Design review of the part built by this model. Coordinates are the model's own, in mm. Coordinates: 2 decimals unless noted, no trailing zeros. Loops run counter-clockwise (first coordinate to the right, second up) from the corner with the lowest first, then second, coordinate; pieces in that order, holes last. Notation, with made-up numbers: M 27,3.5 L 70,3.5 A17 cw 70,12.5 Z; hole C -33.5,19 d4. An arc over 180 degrees is marked long. One line per item, written item: value.
```python
from build123d import *

# Parameters (mm, degrees)
BASE_FLANGE1_DEPTH           = 3.175
SKETCH8_W                    = 12.7
SKETCH8_H                    = 3.175
CUT_EXTRUDE2_DEPTH           = 309.926847379
SKETCH11_R                   = 3.175
CUT_EXTRUDE4_DEPTH           = 309.926847379
SKETCH21_R                   = 2.5527
CUT_EXTRUDE5_DEPTH           = 309.926847379
SKETCH23_W                   = 25.4
SKETCH23_H                   = 3.175
TAB1_DEPTH                   = 3.175
CSK_FOR_M3_SFHCS1_AT_2_COUNT = 2
CSK_FOR_M3_SFHCS1_AT_2_PITCH = 16
CSK_FOR_M3_SFHCS1_AT_3_COUNT = 2
CSK_FOR_M3_SFHCS1_AT_3_PITCH = 27.712812921
CSK_FOR_M3_SFHCS1_AT_4_COUNT = 2
CSK_FOR_M3_SFHCS1_AT_4_PITCH = 32
CSK_FOR_M3_SFHCS1_AT_5_COUNT = 2
CSK_FOR_M3_SFHCS1_AT_5_PITCH = 27.712812921
CSK_FOR_M3_SFHCS1_AT_6_COUNT = 2
CSK_FOR_M3_SFHCS1_AT_6_PITCH = 16


# Sheet-metal steps are written as plain solids
with BuildPart() as part:
    # Sketch1 → Base-Flange1 (new body)
    with BuildSketch(Plane(origin=(0, 0, 0), x_dir=(0, 0, -1), z_dir=(1, 0, 0))):
        with BuildLine():
            Line((0, -80.9625), (0, 80.9625))
            Line((0, 80.9625), (-110.597916699, 80.9625))
            ThreePointArc((-110.597916699, 80.9625), (-137.538685062, 85.883926782), (-160.999479175, 100.0125))
            ThreePointArc((-160.999479175, 100.0125), (-201.559524406, 89.942756121), (-177.8, 55.5625))
            Line((-177.8, 55.5625), (-25.4, 55.5625))
            Line((-25.4, 55.5625), (-25.4, -68.2625))
            Line((-25.4, -68.2625), (-279.4, -68.2625))
            Line((-279.4, -68.2625), (-279.4, -80.9625))
            Line((-279.4, -80.9625), (-228.6, -80.9625))
            Line((-228.6, -80.9625), (-44.45, -131.7625))
            Line((-44.45, -131.7625), (-34.925, -131.7625))
            Line((-34.925, -131.7625), (-34.925, -125.4125))
            Line((-34.925, -125.4125), (-38.1, -125.4125))
            Line((-38.1, -125.4125), (-38.1, -106.3625))
            Line((-38.1, -106.3625), (-6.35, -106.3625))
            Line((-6.35, -106.3625), (-6.35, -125.4125))
            Line((-6.35, -125.4125), (-9.525, -125.4125))
            Line((-9.525, -125.4125), (-9.525, -131.7625))
            Line((-9.525, -131.7625), (0, -131.7625))
            Line((0, -131.7625), (0, -80.9625))
        make_face()
    extrude(amount=-BASE_FLANGE1_DEPTH)

    # Sketch8 → Cut-Extrude2 (cut, through all)
    with BuildSketch(Plane(origin=(0, 0, 0), x_dir=(0, 0, -1), z_dir=(1, 0, 0))):
        with Locations((-19.05, -6.35)):
            Rectangle(SKETCH8_W, SKETCH8_H)
        with Locations((-19.05, -34.925)):
            Rectangle(SKETCH8_W, SKETCH8_H)
    extrude(amount=-CUT_EXTRUDE2_DEPTH, mode=Mode.SUBTRACT)

    # Sketch11 → Cut-Extrude4 (cut, through all)
    with BuildSketch(Plane(origin=(0, 0, 0), x_dir=(0, 0, -1), z_dir=(1, 0, 0))):
        with Locations((-177.8, 80.9625)):
            Circle(SKETCH11_R)
    extrude(amount=-CUT_EXTRUDE4_DEPTH, mode=Mode.SUBTRACT)

    # Sketch21 → Cut-Extrude5 (cut, through all)
    with BuildSketch(Plane(origin=(0, 0, 0), x_dir=(0, 0, -1), z_dir=(1, 0, 0))):
        with Locations((-33.02, -74.6125)):
            Circle(SKETCH21_R)
        with Locations((-106.68, -74.6125)):
            Circle(SKETCH21_R)
        with Locations((-180.34, -74.6125)):
            Circle(SKETCH21_R)
        with Locations((-254, -74.6125)):
            Circle(SKETCH21_R)
        with Locations((-12.7, 61.9125)):
            Circle(SKETCH21_R)
        with Locations((-50.8, 74.6125)):
            Circle(SKETCH21_R)
        with Locations((-88.9, 61.9125)):
            Circle(SKETCH21_R)
    extrude(amount=-CUT_EXTRUDE5_DEPTH, mode=Mode.SUBTRACT)

    # Sketch23 → Tab1 (add)
    with BuildSketch(Plane(origin=(0, 0, 0), x_dir=(0, 0, -1), z_dir=(1, 0, 0))):
        with Locations((-217.17, -66.675)):
            Rectangle(SKETCH23_W, SKETCH23_H)
        with Locations((-143.51, -66.675)):
            Rectangle(SKETCH23_W, SKETCH23_H)
        with Locations((-69.85, -66.675)):
            Rectangle(SKETCH23_W, SKETCH23_H)
    extrude(amount=-TAB1_DEPTH)

    # Sketch25 → CSK for M3 SFHCS1 (revolve, cut)
    with BuildSketch(Plane(origin=(0, 80.9625, 161.8), x_dir=(0, 0, -1), z_dir=(0, 1, 0))):
        Polygon((0, 0), (0, 3.175), (1.7, 3.175), (1.7, 1.66), (3.36, 0), align=None)
    csk_for_m3_sfhcs1 = revolve(axis=Axis((6.35, 80.9625, 161.8), (-1, 0, 0)), mode=Mode.SUBTRACT)

    # CSK for M3 SFHCS1 at 2: CSK for M3 SFHCS1 ×2
    with Locations(*[Vector(0, -0.8660254037844389, 0.4999999999999998) * (i * CSK_FOR_M3_SFHCS1_AT_2_PITCH) for i in range(1, CSK_FOR_M3_SFHCS1_AT_2_COUNT)]):
        add(csk_for_m3_sfhcs1, mode=Mode.SUBTRACT)

    # CSK for M3 SFHCS1 at 3: CSK for M3 SFHCS1 ×2
    with Locations(*[Vector(0, -0.500000000000002, 0.8660254037844376) * (i * CSK_FOR_M3_SFHCS1_AT_3_PITCH) for i in range(1, CSK_FOR_M3_SFHCS1_AT_3_COUNT)]):
        add(csk_for_m3_sfhcs1, mode=Mode.SUBTRACT)

    # CSK for M3 SFHCS1 at 4: CSK for M3 SFHCS1 ×2
    with Locations(*[(0, 0, i * CSK_FOR_M3_SFHCS1_AT_4_PITCH) for i in range(1, CSK_FOR_M3_SFHCS1_AT_4_COUNT)]):
        add(csk_for_m3_sfhcs1, mode=Mode.SUBTRACT)

    # CSK for M3 SFHCS1 at 5: CSK for M3 SFHCS1 ×2
    with Locations(*[Vector(0, 0.5000000000000007, 0.8660254037844384) * (i * CSK_FOR_M3_SFHCS1_AT_5_PITCH) for i in range(1, CSK_FOR_M3_SFHCS1_AT_5_COUNT)]):
        add(csk_for_m3_sfhcs1, mode=Mode.SUBTRACT)

    # CSK for M3 SFHCS1 at 6: CSK for M3 SFHCS1 ×2
    with Locations(*[Vector(0, 0.8660254037844379, 0.5000000000000013) * (i * CSK_FOR_M3_SFHCS1_AT_6_PITCH) for i in range(1, CSK_FOR_M3_SFHCS1_AT_6_COUNT)]):
        add(csk_for_m3_sfhcs1, mode=Mode.SUBTRACT)


solid = part.part
```
(1) Mouldability with a two-part tool opening along Y and no side actions: class faces 1 (the cylindrical face through (-1.57, 85.75, 137.18)), 2 (the cylindrical face through (-1.565, 77.863, 178.488)), 3 (the flat face through (0, -74, 78)), 4 (the cylindrical face through (-1.6, 90.6, 201.3)) as released by +Y, released by -Y, zero draft, split by the parting line, or undercut.
Reply:
face 1: released by +Y
face 2: undercut
face 3: zero draft
face 4: undercut
(2) We need section A-A on z = 116. State the section outline as (x, y) points (1 decimal), then the cut area to 3 significant figures.
Reply:
outline: M -3.2,-112 L 0,-112 L 0,-68.3 L -3.2,-68.3 Z; M -3.2,55.6 L 0,55.6 L 0,81.2 L -3.2,81.2 Z
area: 220 mm2
(3) We need section C-C on z = 240. State the section outline as (x, y) points (1 decimal), then the cut area to 3 significant figures.
Reply:
outline: M -3.2,-81 L 0,-81 L 0,-68.3 L -3.2,-68.3 Z
area: 40.3 mm2
(4) To check wall thickness, follow line 1 along Y through (x, z) = (-0.9, 180.34); line 2 along Y through (x, z) = (-2.55, 185.8); line 3 along Z through (x, y) = (-2.8, 67.5). State the ranges of each line that lie inside material, in increasing order. Write a range as [from, to].
Reply:
line 1: y = [-94.28, -77.17], [-72.06, -68.26], [55.69, 79.06], [82.87, 106.24]
line 2: y = [-92.77, -68.26], [56.86, 65.41], [68.81, 93.12], [96.52, 105.07]
line 3: z = [0, 168.15], [171.45, 184.15], [187.45, 199.34]
(5) Insertion check: pin 1 (1.6 mm diameter, centred on x = -1, y = -7, fed in from +Z); pin 2 (1 mm diameter, centred on x = -1.5, z = 24, fed in from -Y); pin 3 (1.6 mm diameter, centred on x = -2, z = 37.5, fed in from +Y); pin 4 (4 mm diameter, centred on y = -74.61, z = 254, fed in from +X). Each pin has a flat end and moves straight along its axis. Give the tip position at first contact, or say it passes through.
Reply:
pin 1: stops at z = 12.7
pin 2: stops at y = -106.36
pin 3: stops at y = 80.96
pin 4: passes through
(6) We need section B-B on y = 3. State the section outline as (x, z) points (3 decimals).
Reply:
outline: M -3.175,0 L 0,0 L 0,25.4 L -3.175,25.4 Z
